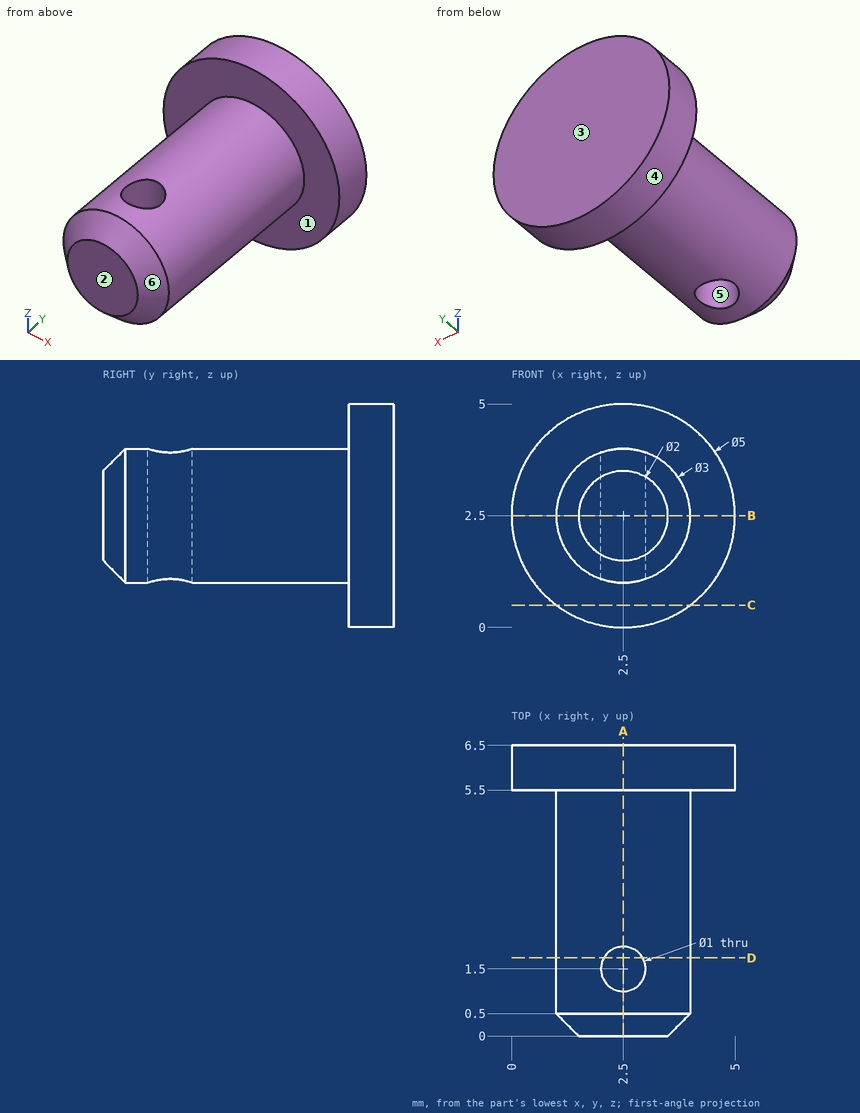
Job drawing, mm, ordinate dimensions from the low corner. One solid piece. A direction names the side the tool comes from. Coordinates: 2 decimals unless noted, no trailing zeros. Write each loop counter-clockwise with the first axis right and the second up, starting at its lowest first coordinate (ties: lowest second). Pieces come first, ordered by that corner, then holes.
Item 1: Pin check, flat tips, straight feed: pin 1 (1.5 mm diameter, centred on x = 1.5, y = 4, fed in from -Z); pin 2 (3 mm diameter, centred on x = 1.5, z = 4.5, fed in from -Y). Stop position of each tip, or through.
Item 2: Slice it at B-B (z = 2.5). Write the cut outline in (x, y).
Item 3: Probe line 1 (Y direction, x = 2.5, z = 3.1); line 2 (X direction, y = 1.5, z = 3.1); line 3 (Y direction, x = 1.8, z = 0.55). List the from-to ranges inside material, lowest first.
Item 4: Mould opens along Y. For the marked faces 3, 4, 5 and 6 say: released by +Y, released by -Y, zero draft, split by the parting line, or undercut.
Item 5: Which spindle directions (+Z, -Z, +X, -X, +Y, -Y) get a long thin tool onto all of the face, cutting with end or side? Do the marked faces 1 and 2. Say none if no direction does.
Item 6: Slice it at D-D (y = 1.75). Write the cut outline in (x, z), and give its area (3 significant figures).
Item 7: Slice it at C-C (z = 0.5). Write the cut outline in (x, y), and give its area (3 significant figures).
Item 8: Slice it at A-A (x = 2.5). Write the cut outline in (y, z), and give its area (4 significant figures).
Results found:
1. pin 1: stops at z = 1.02
1. pin 2: stops at y = 0
2. outline: (0, 5.5) - (1, 5.5) - (1, 0.5) - (1.5, 0) - (3.5, 0) - (4, 0.5) - (4, 5.5) - (5, 5.5) - (5, 6.5) - (0, 6.5) - close; hole circle Ø1 at (2.5, 1.5)
3. line 1: y = 0 to 1, 2 to 6.5
3. line 2: x = 1.13 to 2, 3 to 3.87
3. line 3: y = 5.5 to 6.5
4. face 3: released by +Y
4. face 4: zero draft
4. face 5: undercut
4. face 6: released by -Y
5. face 1: -Y
5. face 2: +Z, -Z, +X, -X, -Y
6. outline: (2.07, 1.06) - (2.07, 3.94) arc R1.5 ccw to start; (2.93, 1.06) arc R1.5 ccw to (2.93, 3.94) - close
6. area: 4.51 mm2
7. outline: (1, 5.5) - (4, 5.5) - (4, 6.5) - (1, 6.5) - close
7. area: 3.00 mm2
8. outline: (0, 1.5) - (0.5, 1) - (1, 1) - (1, 4) - (0.5, 4) - (0, 3.5) - close; (2, 1) - (5.5, 1) - (5.5, 0) - (6.5, 0) - (6.5, 5) - (5.5, 5) - (5.5, 4) - (2, 4) - close
8. area: 18.25 mm2
